Input: dimensioned drawing with shaded views. Units: mm. Origin: part minimum x, y, z. A direction names the side the tool comes from. Round coordinates to 2 decimals unless told otherwise and drop trailing zeros. Loops run counter-clockwise (first coordinate to the right, second up) from the corner with the lowest first, then second, coordinate; pieces in that order, holes last. Notation, with made-up numbers: (67.5, -35) -> (106.5, -35) arc R27 cw to (106.5, -2) -> close; hole circle Ø5 at (-29.75, -36). An arc over 180 degrees is marked (long way). Answer as a JSON object with one key per item and string values.
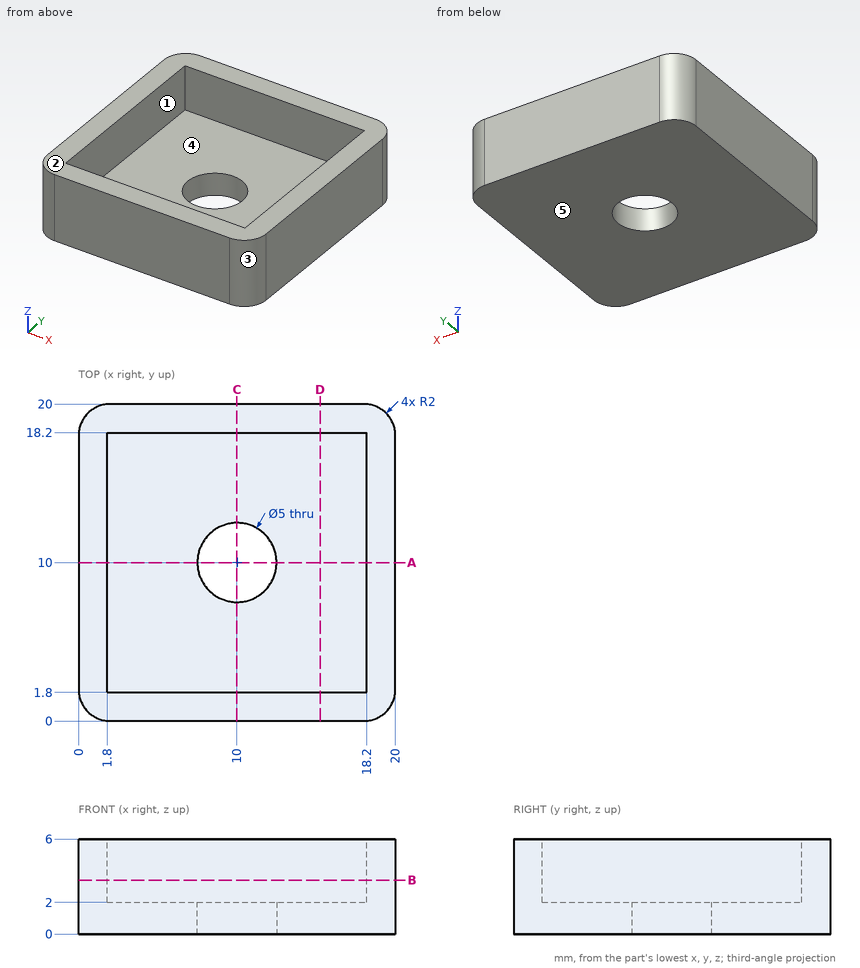
1) Reachability of the marked faces 4 and 5 from +Z, -Z, +X, -X, +Y, -Y: full face, straight path, thin tool, end or side. Return the list, or none.
Output:
{"face 4": "+Z", "face 5": "-Z, +X, -X, +Y, -Y"}
2) Ray query, probe 1 along Y at (x, z) = (10, 1.5); probe 2 along Y at (x, z) = (6, 4.05). Return the intervals inside material, ascending.
Output:
{"probe 1": "y = 0 to 7.5, 12.5 to 20", "probe 2": "y = 0 to 1.8, 18.2 to 20"}
3) Section A-A, the plane y = 10. Output: boundary loops of the cut face in (x, z), plus the area to 3 significant figures.
Output:
{"outline": "(0, 0) -> (7.5, 0) -> (7.5, 2) -> (1.8, 2) -> (1.8, 6) -> (0, 6) -> close; (12.5, 0) -> (20, 0) -> (20, 6) -> (18.2, 6) -> (18.2, 2) -> (12.5, 2) -> close", "area": "44.4 mm^2"}
4) Draft query along Y for the marked faces 1, 2 and 3. Return one class per face: +Y half, -Y half, draft (parallel to the pull), parting line (faces both ways), or undercut.
Output:
{"face 1": "undercut", "face 2": "draft", "face 3": "-Y half"}
5) Section D-D, the plane x = 15.25. Output: boundary loops of the cut face in (y, z), plus the area to 3 significant figures.
Output:
{"outline": "(0, 0) -> (20, 0) -> (20, 6) -> (18.2, 6) -> (18.2, 2) -> (1.8, 2) -> (1.8, 6) -> (0, 6) -> close", "area": "54.4 mm^2"}
6) Contact query for a flat-ended pin moving along its axis: P1, Ø8, axis at x = 7.5, y = 7.5, coming from the +Z side. Output: stop coordinate, or through.
Output:
{"P1": "stops at z = 2"}
7) Section B-B, the plane z = 3.4. Output: boundary loops of the cut face in (x, y), plus the area to 3 significant figures.
Output:
{"outline": "(0, 2) arc R2 ccw to (2, 0) -> (18, 0) arc R2 ccw to (20, 2) -> (20, 18) arc R2 ccw to (18, 20) -> (2, 20) arc R2 ccw to (0, 18) -> close; hole (1.8, 1.8) -> (18.2, 1.8) -> (18.2, 18.2) -> (1.8, 18.2) -> close", "area": "128 mm^2"}
